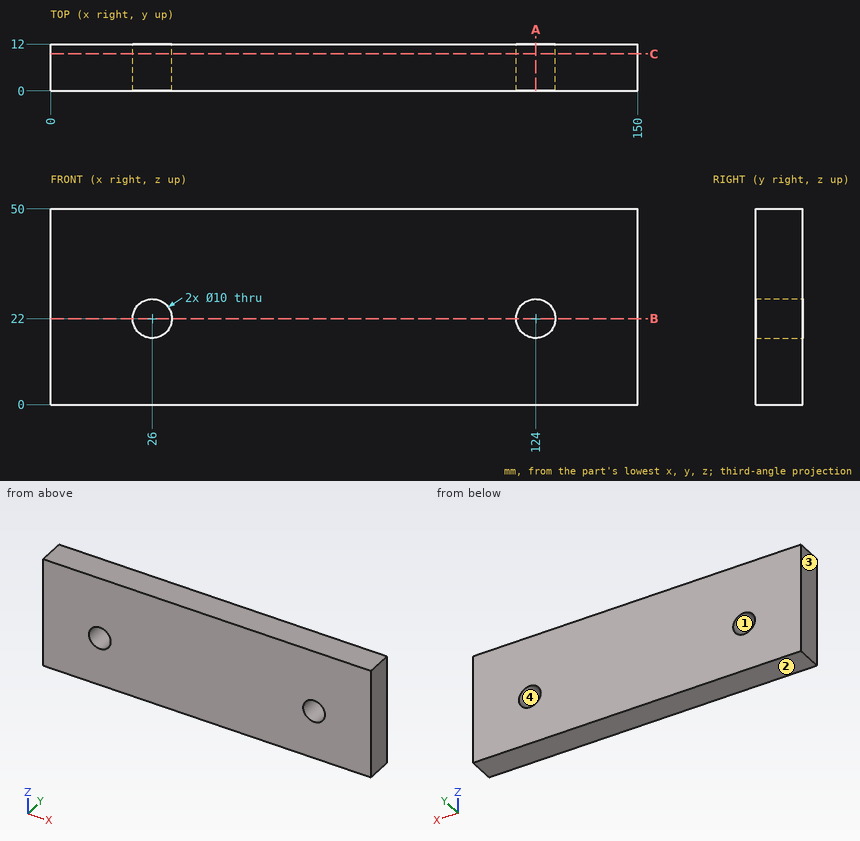
Answer from the drawing. Dimensions are ordinates in mm from the lowest x, y and z of the part. Coordinates: 2 decimals unless noted, no trailing zeros. Loops run counter-clockwise (first coordinate to the right, second up) from the corner with the lowest first, then second, coordinate; pieces in that order, holes last. Notation, with made-up numbers: (33.25, -28) -> (46.25, -28) arc R4 ccw to (46.25, -21) -> close; hole circle Ø11 at (-25, 6.5). An arc over 180 degrees is marked (long way). Answer as CSV lines item,"result".
Q1. The part is cut by section A-A on x = 124. Write down the section's boundary in (y, z), and give its area (3 significant figures).
Findings:
outline,"(0, 0) -> (12, 0) -> (12, 17) -> (0, 17) -> close; (0, 27) -> (12, 27) -> (12, 50) -> (0, 50) -> close"
area,"480 mm²"
Q2. Find the intervals of material crossed by probe 1 along Z at (x, y) = (26, 9); probe 2 along X at (y, z) = (9.25, 23); probe 3 along Z at (x, y) = (25, 1.5), in increasing order.
Findings:
probe 1,"z = 0 to 17, 27 to 50"
probe 2,"x = 0 to 21.1, 30.9 to 119.1, 128.9 to 150"
probe 3,"z = 0 to 17.1, 26.9 to 50"
Q3. For a pull along X with two mould halves and no side action, classify the marked faces 1, 2, 3 and 4 as +X half, -X half, draft (parallel to the pull), parting line (faces both ways), or undercut.
Findings:
face 1,"undercut"
face 2,"draft"
face 3,"-X half"
face 4,"undercut"
Q4. This flat-tipped pin is pushed along its axis until it touches: pin 1 (8 mm diameter, centred on x = 124, z = 22, fed in from +Y). Where does it stop, or does it pass through?
Findings:
pin 1,"passes through"
Q5. The part is cut by section B-B on z = 22. Write down the section's boundary in (x, y).
Findings:
outline,"(0, 0) -> (21, 0) -> (21, 12) -> (0, 12) -> close; (31, 0) -> (119, 0) -> (119, 12) -> (31, 12) -> close; (129, 0) -> (150, 0) -> (150, 12) -> (129, 12) -> close"
Q6. The part is cut by section C-C on y = 9.5. Write down the section's boundary in (x, z), and give its area (3 significant figures).
Findings:
outline,"(0, 0) -> (150, 0) -> (150, 50) -> (0, 50) -> close; hole circle Ø10 at (26, 22); hole circle Ø10 at (124, 22)"
area,"7,340 mm²"
